from build123d import *

# Parameters (mm, degrees)
SKETCH1_R           = 38.1
BOSS_EXTRUDE1_DEPTH = 1.27
BOSS_EXTRUDE2_DEPTH = 1.27
SKETCH3_R           = 7.366
CUT_EXTRUDE1_DEPTH  = 10
CIRPATTERN1_COUNT   = 18
SKETCH4_R           = 25.4
CUT_EXTRUDE2_DEPTH  = 0.254


with BuildPart() as part:
    # Sketch1 → Boss-Extrude1 (new body)
    with BuildSketch(Plane.XY):
        Circle(SKETCH1_R)
    extrude(amount=BOSS_EXTRUDE1_DEPTH)

    # Sketch2 → Boss-Extrude2 (add)
    with BuildSketch(Plane.XY.offset(1.27)):
        with BuildLine():
            Line((-1.27, 44.45), (1.27, 44.45))
            Line((1.27, 44.45), (4.347073366, 37.851194871))
            ThreePointArc((4.347073366, 37.851194871), (0, 38.1), (-4.347073366, 37.851194871))
            Line((-4.347073366, 37.851194871), (-1.27, 44.45))
        make_face()
    boss_extrude2 = extrude(amount=-BOSS_EXTRUDE2_DEPTH)

    # Sketch3 → Cut-Extrude1 (cut)
    with BuildSketch(Plane(origin=(0, 0, 0), x_dir=(-1, 0, 0), z_dir=(0, 0, -1))):
        Circle(SKETCH3_R)
    extrude(amount=-CUT_EXTRUDE1_DEPTH, mode=Mode.SUBTRACT)

    # CirPattern1: Boss-Extrude2 ×18 about axis
    cirpattern1_axis = Axis((0, 0, 0), (0, 0, 1))
    for i in range(1, CIRPATTERN1_COUNT):
        add(boss_extrude2.rotate(cirpattern1_axis, i * 360 / CIRPATTERN1_COUNT))

    # Sketch4 → Cut-Extrude2 (cut)
    with BuildSketch(Plane(origin=(0, 0, 0), x_dir=(-1, 0, 0), z_dir=(0, 0, -1))):
        Circle(SKETCH4_R)
    extrude(amount=-CUT_EXTRUDE2_DEPTH, mode=Mode.SUBTRACT)


solid = part.part
Can you work these out from the model? Positions are in its coordinate system, mm. A direction names the side the tool comes from. Give positions to 0.01 mm unless a question says otherwise; leave off trailing zeros. Loops run counter-clockwise (first coordinate to the right, second up) from the corner with the lowest first, then second, coordinate; pieces in that order, holes last. Notation, with made-up numbers: (66, 60) - (94, 60) arc R14 ccw to (94, 76) - close; hole circle Ø8 at (30.25, -35). An arc over 180 degrees is marked (long way). Answer as a JSON object with one key per item and string values.
Q1. Imagine slicing it at C-C on y = 39. Write out the boundary of the cut face in (x, z), plus the area to 3 significant figures.
Geometry says:
{"outline": "(-16.6, 0) - (-10.81, 0) - (-10.81, 1.27) - (-16.6, 1.27) - close; (-3.81, 0) - (3.81, 0) - (3.81, 1.27) - (-3.81, 1.27) - close; (10.81, 0) - (16.6, 0) - (16.6, 1.27) - (10.81, 1.27) - close", "area": "24.4 mm²"}
Q2. If we mould it in two halves opening along Y, with no side actions, what happens to faces 1 (the flat face through (40.087, -9.898, 0.644)), 2 (the cylindrical face through (19.022, -33.012, 0.626)), 3 (the cylindrical face through (19.08, 32.98, 0.63)), 4 (the flat face through (41.055, 4.409, 0.644))? For each: pulls with the +Y half, pulls with the -Y half, needs draft (parallel to the pull), parting line crosses it, or undercut.
Geometry says:
{"face 1": "undercut", "face 2": "pulls with the -Y half", "face 3": "pulls with the +Y half", "face 4": "undercut"}
Q3. Imagine slicing it at D-D on x = 32. Write out the boundary of the cut face in (y, z), plus the area to 3 significant figures.
Geometry says:
{"outline": "(-22.81, 0) - (22.81, 0) - (22.81, 1.27) - (-22.81, 1.27) - close", "area": "57.9 mm²"}
Q4. Which directions (+Z, -Z, +X, -X, +Y, -Y) give clear straight access to the entire face, cutting with the end or side of a thin tool? Please do faces 5 (the cylindrical face through (-19.022, 33.012, 0.626)), 6 (the flat face through (39.988, 9.925, 0.644)), 7 (the flat face through (-5, 6, 0.254)), 8 (the flat face through (-2.787, -41.197, 0.644)).
Geometry says:
{"face 5": "+Z, -Z, +Y", "face 6": "+Z, -Z, +X", "face 7": "-Z", "face 8": "+Z, -Z, -Y"}
Q5. Imagine slicing it at B-B on x = 0. Write out the boundary of the cut face in (y, z), plus the area to 3 significant figures.
Geometry says:
{"outline": "(-44.45, 0) - (-25.4, 0) - (-25.4, 0.25) - (-7.37, 0.25) - (-7.37, 1.27) - (-44.45, 1.27) - close; (7.37, 0.25) - (25.4, 0.25) - (25.4, 0) - (44.45, 0) - (44.45, 1.27) - (7.37, 1.27) - close", "area": "85.0 mm²"}
Q6. Imagine slicing it at A-A on y = 0. Write out the boundary of the cut face in (x, z), plus the area to 3 significant figures.
Geometry says:
{"outline": "(-38.1, 0) - (-25.4, 0) - (-25.4, 0.25) - (-7.37, 0.25) - (-7.37, 1.27) - (-38.1, 1.27) - close; (7.37, 0.25) - (25.4, 0.25) - (25.4, 0) - (38.1, 0) - (38.1, 1.27) - (7.37, 1.27) - close", "area": "68.9 mm²"}
Q7. If I drill on L1, parallel to Y at x = 0, z = 1.05; L2, parallel to X at y = 40, z = 0.65; L3, parallel to X at y = 33, z = 0.7, over which ranges is the centre line in solid material (lowest first)?
Geometry says:
{"L1": "-44.45 to -7.37, 7.37 to 44.45", "L2": "-16.51 to -11.81, -3.35 to 3.35, 11.81 to 16.51", "L3": "-29.48 to -23.6, -19.04 to 19.04, 23.6 to 29.48"}
Q8. Will this pin go through, and if not, where does the flat tip stop? P1, Ø9, axis at x = 0, y = 0, coming from the +Z side (3 decimals).
Geometry says:
{"P1": "through"}
